```python
from build123d import *

# Parameters (mm, degrees)
SKETCH1_W           = 121.92
SKETCH1_H           = 99.06
BOSS_EXTRUDE1_DEPTH = 2
SKETCH2_R           = 2.371054243
CUT_EXTRUDE1_DEPTH  = 2
SKETCH3_W           = 25
SKETCH3_H           = 15
BOSS_EXTRUDE2_DEPTH = 6
SKETCH4_W           = 12.871437318
SKETCH4_H           = 17.274823769
BOSS_EXTRUDE3_DEPTH = 15


with BuildPart() as part:
    # Sketch1 → Boss-Extrude1 (new body)
    with BuildSketch(Plane(origin=(0, 0, 0), x_dir=(1, 0, 0), z_dir=(0, 1, 0))):
        Rectangle(SKETCH1_W, SKETCH1_H)
    extrude(amount=BOSS_EXTRUDE1_DEPTH)

    # Sketch2 → Cut-Extrude1 (cut)
    with BuildSketch(Plane(origin=(0, 2, 0), x_dir=(1, 0, 0), z_dir=(0, 1, 0))):
        with Locations((-55.88, 44.45)):
            Circle(SKETCH2_R)
        with Locations((55.88, 44.45)):
            Circle(SKETCH2_R)
        with Locations((55.88, -44.45)):
            Circle(SKETCH2_R)
        with Locations((-55.88, -44.45)):
            Circle(SKETCH2_R)
    extrude(amount=-CUT_EXTRUDE1_DEPTH, mode=Mode.SUBTRACT)

    # Sketch3 → Boss-Extrude2 (add)
    with BuildSketch(Plane(origin=(0, 2, 0), x_dir=(1, 0, 0), z_dir=(0, 1, 0))):
        with Locations((-36.106611978, 36.968817018)):
            Rectangle(SKETCH3_W, SKETCH3_H)
        with Locations((36.106611978, 36.968817018)):
            Rectangle(SKETCH3_W, SKETCH3_H)
    extrude(amount=BOSS_EXTRUDE2_DEPTH)

    # Sketch4 → Boss-Extrude3 (add)
    with BuildSketch(Plane(origin=(0, 2, 0), x_dir=(1, 0, 0), z_dir=(0, 1, 0))):
        with Locations((-54.026164533, -17.274823769)):
            Rectangle(SKETCH4_W, SKETCH4_H)
    extrude(amount=BOSS_EXTRUDE3_DEPTH)


solid = part.part
```
Geometry check sheet. Reference: the model listing, model coordinates, mm. A direction names the side the tool comes from. Round coordinates to 2 decimals unless told otherwise and drop trailing zeros. Order: outer loops, then holes, each group sorted by start corner. A loop starts at its lowest first (then second) coordinate and runs counter-clockwise, first axis right, second up. Notation, with made-up numbers: (62, 63.5) - (73, 63.5) arc R18 ccw to (73, 68.5) - close; hole circle Ø6 at (79.5, 14.5). An arc over 180 degrees is marked (long way). Use a Markdown table: item, result. Add a question column.
(1) Material ranges on line 1 along Z through (x, y) = (55.88, 0.8); line 2 along X through (y, z) = (1.6, -44.45); line 3 along X through (y, z) = (4, 14.5), recorded low to high. Write a range as [from, to].
(2) Sectioned sample at D-D, the plane y = 13. Enter the section's corners in (x, z), and give its area (3 significant figures).
(3) Sectioned sample at B-B, the plane x = 55.88. Enter the section's corners in (y, z).
(4) Depth check by flat-ended pin: pin 1 (1.8 mm diameter, centred on x = -35.5, y = 4.5, fed in from -Z); pin 2 (7.5 mm diameter, centred on x = 55.88, z = -44.45, fed in from +Y); pin 3 (7.5 mm diameter, centred on x = -33, z = -36.5, fed in from +Y); pin 4 (4.5 mm diameter, centred on x = -55.88, z = 44.45, fed in from +Y). Enter the tip coordinate at first touch or a pass-through.
(5) Release check for a two-part mould opening along Z. For faces 4 (the flat face through (23.607, 5, -37)), 5 (the cylindrical face through (57.15, 1.01, -46.45)), 6 (the flat face through (-36, 5, -44.469)) record: pulls with the +Z half, pulls with the -Z half, needs draft (parallel to the pull), parting line crosses it, or undercut.
(6) Sectioned sample at A-A, the plane z = 44.45. Enter the section's corners in (x, y).
(7) Tool access check on faces 1 (the flat face through (36, 5, -44.469)), 2 (the flat face through (-47.59, 9, 17)), 3 (the flat face through (-48.607, 5, -37)). Record the directions out of +Z, -Z, +X, -X, +Y, -Y that give a thin tool (end or side, any length) a straight path to the whole face; none if there is none.
(8) Sectioned sample at C-C, the plane z = -31.5. Enter the section's corners in (x, y).
Answers below:
| question | item | result |
|---|---|---|
| 1 | line 1 | [-49.53, -46.82], [-42.08, 42.08], [46.82, 49.53] |
| 1 | line 2 | [-60.96, -58.25], [-53.51, 53.51], [58.25, 60.96] |
| 1 | line 3 | [-60.46, -47.59] |
| 2 | outline | (-60.46, 8.64) - (-47.59, 8.64) - (-47.59, 25.91) - (-60.46, 25.91) - close |
| 2 | area | 222 mm² |
| 3 | outline | (0, -49.53) - (2, -49.53) - (2, -46.82) - (0, -46.82) - close; (0, -42.08) - (2, -42.08) - (2, 42.08) - (0, 42.08) - close; (0, 46.82) - (2, 46.82) - (2, 49.53) - (0, 49.53) - close |
| 4 | pin 1 | z = -44.47 |
| 4 | pin 2 | y = 2 |
| 4 | pin 3 | y = 8 |
| 4 | pin 4 | through |
| 5 | face 4 | needs draft |
| 5 | face 5 | undercut |
| 5 | face 6 | pulls with the -Z half |
| 6 | outline | (-60.96, 0) - (-58.25, 0) - (-58.25, 2) - (-60.96, 2) - close; (-53.51, 0) - (53.51, 0) - (53.51, 2) - (-53.51, 2) - close; (58.25, 0) - (60.96, 0) - (60.96, 2) - (58.25, 2) - close |
| 7 | face 1 | -Z, +X, -X, +Y |
| 7 | face 2 | +Z, +X, +Y |
| 7 | face 3 | -Z, -X, +Y |
| 8 | outline | (-60.96, 0) - (60.96, 0) - (60.96, 2) - (48.61, 2) - (48.61, 8) - (23.61, 8) - (23.61, 2) - (-23.61, 2) - (-23.61, 8) - (-48.61, 8) - (-48.61, 2) - (-60.96, 2) - close |
